from build123d import *

# Parameters (mm, degrees)
BOSS_EXTRUDE1_DEPTH                              = 10
F_2_5_2_5_DIAMETER_HOLE1_D                       = 2.5
F_2_5_2_5_DIAMETER_HOLE1_DEPTH                   = 10
F_2_5_2_5_DIAMETER_HOLE1_TIP                     = 1.25
CBORE_FOR_M5_HEX_HEAD_MACHINE_SCREW2_D           = 4.25
CBORE_FOR_M5_HEX_HEAD_MACHINE_SCREW2_DEPTH       = 5
CBORE_FOR_M5_HEX_HEAD_MACHINE_SCREW2_CBORE_D     = 5
CBORE_FOR_M5_HEX_HEAD_MACHINE_SCREW2_CBORE_DEPTH = 0.5
CBORE_FOR_M5_HEX_HEAD_MACHINE_SCREW2_TIP         = 1.276828815
M3_CLEARANCE_HOLE1_D                             = 3.4
M3_CLEARANCE_HOLE1_DEPTH                         = 5
M3_CLEARANCE_HOLE1_TIP                           = 1.021463052
FILLET1_R                                        = 4
CHAMFER1_SIZE                                    = 0.75


with BuildPart() as part:
    # Sketch1 → Boss-Extrude1 (new, symmetric)
    with BuildSketch(Plane.XY):
        with BuildLine():
            Line((6.5, -25.491610633), (6.5, -15.491610633))
            ThreePointArc((6.5, -15.491610633), (4.047863744, -16.305054404), (1.5, -16.732901721))
            Line((1.5, -16.732901721), (1.5, -25.491610633))
            Line((1.5, -25.491610633), (6.5, -25.491610633))
        make_face()
        with BuildLine():
            ThreePointArc((-1.5, -16.732901721), (-4.047863744, -16.305054404), (-6.5, -15.491610633))
            Line((-6.5, -15.491610633), (-6.5, -25.491610633))
            Line((-6.5, -25.491610633), (-1.5, -25.491610633))
            Line((-1.5, -25.491610633), (-1.5, -16.732901721))
        make_face()
        with BuildLine():
            Line((-16.8, 21.8), (-16.8, 0))
            ThreePointArc((-16.8, 0), (-13.989996426, -9.301612763), (-6.5, -15.491610633))
            ThreePointArc((-6.5, -15.491610633), (-4.047863744, -16.305054404), (-1.5, -16.732901721))
            Line((-1.5, -16.732901721), (-1.5, -11.704272724))
            ThreePointArc((-1.5, -11.704272724), (-7.795511529, 8.858329414), (11.8, 0))
            ThreePointArc((11.8, 0), (8.858329414, -7.795511529), (1.5, -11.704272724))
            Line((1.5, -11.704272724), (1.5, -16.732901721))
            ThreePointArc((1.5, -16.732901721), (4.047863744, -16.305054404), (6.5, -15.491610633))
            ThreePointArc((6.5, -15.491610633), (13.989996426, -9.301612763), (16.8, 0))
            Line((16.8, 0), (16.8, 21.8))
            Line((16.8, 21.8), (-16.8, 21.8))
        make_face()
    extrude(amount=BOSS_EXTRUDE1_DEPTH, both=True)

    # Ø2.5 (2.5) Diameter Hole1
    with Locations(Plane(origin=(0, 21.8, 0), x_dir=(1, 0, 0), z_dir=(0, 1, 0))):
        with Locations((-11.8, -5), (-11.8, 5), (11.8, 5), (11.8, -5)):
            Hole(F_2_5_2_5_DIAMETER_HOLE1_D / 2, depth=F_2_5_2_5_DIAMETER_HOLE1_DEPTH)
            with Locations((0, 0, -(F_2_5_2_5_DIAMETER_HOLE1_DEPTH + F_2_5_2_5_DIAMETER_HOLE1_TIP / 2))):  # 90° drill point
                Cone(0, F_2_5_2_5_DIAMETER_HOLE1_D / 2, F_2_5_2_5_DIAMETER_HOLE1_TIP, mode=Mode.SUBTRACT)

    # CBORE for M5 Hex Head Machine Screw2
    with Locations(Plane(origin=(6.5, 0, 0), x_dir=(0, 0, -1), z_dir=(1, 0, 0))):
        with Locations((5, -20.491610633), (-5, -20.491610633)):
            CounterBoreHole(CBORE_FOR_M5_HEX_HEAD_MACHINE_SCREW2_D / 2, CBORE_FOR_M5_HEX_HEAD_MACHINE_SCREW2_CBORE_D / 2, CBORE_FOR_M5_HEX_HEAD_MACHINE_SCREW2_CBORE_DEPTH, depth=CBORE_FOR_M5_HEX_HEAD_MACHINE_SCREW2_DEPTH)
            with Locations((0, 0, -(CBORE_FOR_M5_HEX_HEAD_MACHINE_SCREW2_DEPTH + CBORE_FOR_M5_HEX_HEAD_MACHINE_SCREW2_TIP / 2))):  # 118° drill point
                Cone(0, CBORE_FOR_M5_HEX_HEAD_MACHINE_SCREW2_D / 2, CBORE_FOR_M5_HEX_HEAD_MACHINE_SCREW2_TIP, mode=Mode.SUBTRACT)

    # M3 Clearance Hole1
    with Locations(Plane.ZY.offset(6.5)):
        with Locations((-5, -20.491610633), (5, -20.491610633)):
            Hole(M3_CLEARANCE_HOLE1_D / 2, depth=M3_CLEARANCE_HOLE1_DEPTH)
            with Locations((0, 0, -(M3_CLEARANCE_HOLE1_DEPTH + M3_CLEARANCE_HOLE1_TIP / 2))):  # 118° drill point
                Cone(0, M3_CLEARANCE_HOLE1_D / 2, M3_CLEARANCE_HOLE1_TIP, mode=Mode.SUBTRACT)

    # Fillet1
    fillet1_edges = [part.edges().sort_by_distance(p)[0] for p in [
        (1.5, -11.704272724, 0),
        (-1.5, -11.704272724, 0),
        (-6.5, -15.491610633, 0),
        (6.5, -15.491610633, 0),
    ]]
    fillet(fillet1_edges, radius=FILLET1_R)

    # Chamfer1
    chamfer1_edges = [part.edges().sort_by_distance(p)[0] for p in [
        (-16.8, 21.8, 0),
        (16.8, 21.8, 0),
    ]]
    chamfer(chamfer1_edges, length=CHAMFER1_SIZE)


solid = part.part
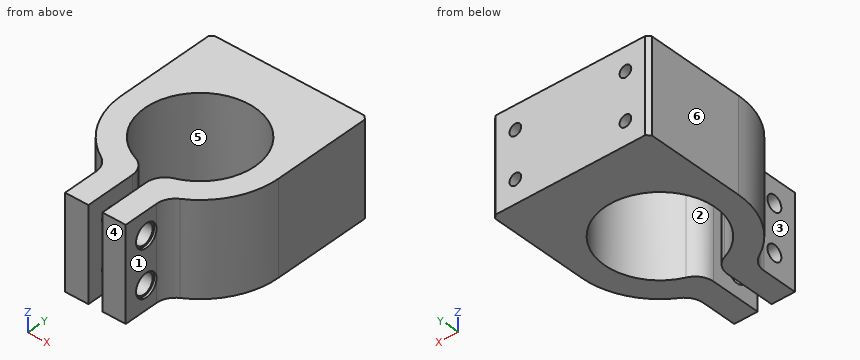
Design review of the part built by this model. Coordinates are the model's own, in mm. Face numbers are marked on the shaded views. A direction names the side the tool comes from. Round coordinates to 2 decimals unless told otherwise and drop trailing zeros. Loops run counter-clockwise (first coordinate to the right, second up) from the corner with the lowest first, then second, coordinate; pieces in that order, holes last. Notation, with made-up numbers: (81.25, -17.5) - (110.25, -17.5) arc R30 ccw to (110.25, 8.5) - close; hole circle Ø3 at (41, 67.25). An arc over 180 degrees is marked (long way). One line per item, written item: value. Start each with the question number.
1) Insertion check: pin 1 Ø10 at (x, z) = (-13, 4) entering from -Y; pin 2 Ø3 at (y, z) = (-19, -0.5) entering from -X; pin 3 Ø4 at (y, z) = (-19.5, -4) entering from +X. Each pin has a flat end and moves straight along its axis. Give the tip position at first contact, or say it passes through.
2) Draft analysis for pull direction Y (two halves, no side actions). For the marked faces 4, 5 and 6, state which applies: +Y half, -Y half, draft (parallel to the pull), parting line (faces both ways), or undercut.
3) To check wall thickness, follow L1, parallel to Y at x = -3.7, z = -5; L2, parallel to Y at x = -4.8, z = -5; L3, parallel to X at y = -18, z = 6.25. State the ranges of each line that lie inside material, in increasing order. Write a range as from..to.
4) For the marked faces 1, 2 and 3, list the 3-axis set-ups (+Z, -Z, +X, -X, +Y, -Y) from which the entire face can be reached by the end or side of a thin tool; tool diameter is ignored.
5) Consider section A-A on y = 13.5. Give the boundary of the cut face in (x, z).
6) Consider section C-C on z = 8.75. Give the boundary of the cut face in (x, y).
7) Consider section B-B on y = 6.5. Give the boundary of the cut face in (x, z).
8) Consider section D-D on x = 0. Give the boundary of the cut face in (y, z).
Reported:
1. pin 1: stops at y = -14.83
1. pin 2: stops at x = -6.53
1. pin 3: stops at x = 6.53
2. face 4: -Y half
2. face 5: undercut
2. face 6: draft
3. L1: y = -25.49..-22.19, -18.79..-11.24, 11.2..21.8
3. L2: y = -25.49..-22.19, -18.79..-10.78, 10.78..21.8
3. L3: x = -6.5..-1.5, 1.5..6.5
4. face 1: +Z, -Z, +X, -Y
4. face 2: +Z, -Z
4. face 3: +Z, -Z, -X, -Y
5. outline: (-16.8, -10) - (16.8, -10) - (16.8, 10) - (-16.8, 10) - close; hole circle Ø2.5 at (-11.8, -5); hole circle Ø2.5 at (-11.8, 5); hole circle Ø2.5 at (11.8, -5); hole circle Ø2.5 at (11.8, 5)
6. outline: (-16.8, 0) arc R16.8 ccw to (-8.48, -14.5) arc R4 cw to (-6.5, -17.96) - (-6.5, -25.49) - (-1.5, -25.49) - (-1.5, -14.81) arc R4 ccw to (-4.11, -11.06) arc R11.8 cw (long way) to (4.11, -11.06) arc R4 ccw to (1.5, -14.81) - (1.5, -25.49) - (6.5, -25.49) - (6.5, -17.96) arc R4 cw to (8.48, -14.5) arc R16.8 ccw to (16.8, 0) - (16.8, 21.05) - (16.05, 21.8) - (-16.05, 21.8) - (-16.8, 21.05) - close
7. outline: (-16.8, -10) - (-9.85, -10) - (-9.85, 10) - (-16.8, 10) - close; (9.85, -10) - (16.8, -10) - (16.8, 10) - (9.85, 10) - close
8. outline: (11.8, -10) - (21.8, -10) - (21.8, 10) - (11.8, 10) - close
